Source: CAD feature listing. Evaluate the final solid. Frame: model axes, mm. Face numbers are marked on the shaded views. A direction names the side the tool comes from. Coordinates: 2 decimals unless noted, no trailing zeros. Loops run counter-clockwise (first coordinate to the right, second up) from the corner with the lowest first, then second, coordinate; pieces in that order, holes last. Notation, with made-up numbers: (12.25, -10.5) -> (64.25, -10.5) arc R15 ccw to (64.25, 11.5) -> close; hole circle Ø1 at (21.25, -32.75). An arc over 180 degrees is marked (long way). Answer as a JSON object with one key per item and string values. Group by question number.
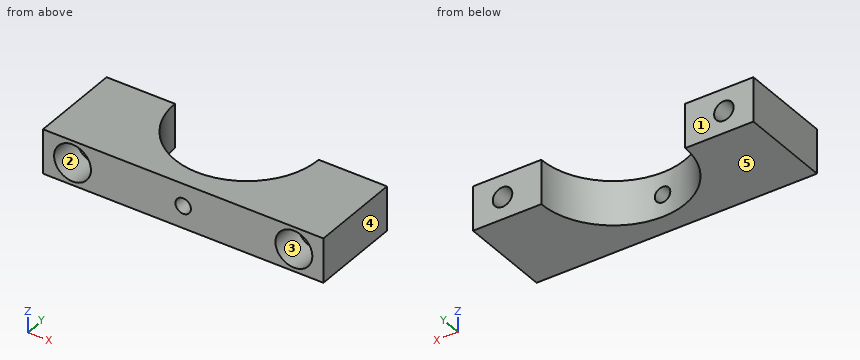
from build123d import *

# Parameters (mm, degrees)
SKETCH_1_W                = 76
SKETCH_1_H                = 12
EXTRUDE_1_DEPTH           = 25
CUT_EXTRUDE_1_REACH       = 49.043
SKETCH_2_R                = 19.5
HOLE_WIZARD_M5_1_D        = 4.2
HOLE_WIZARD_1_D           = 5.3
HOLE_WIZARD_1_CBORE_D     = 10
HOLE_WIZARD_1_CBORE_DEPTH = 8.7


with BuildPart() as part:
    # 草图1 → 凸台-拉伸1 (new body)
    with BuildSketch(Plane(origin=(0, 0, 0), x_dir=(1, 0, 0), z_dir=(0, 1, 0))):
        Rectangle(SKETCH_1_W, SKETCH_1_H)
    extrude(amount=-EXTRUDE_1_DEPTH)

    # 草图2 → 切除-拉伸1 (cut, up to next)
    with BuildSketch(Plane.XY.offset(6), mode=Mode.PRIVATE) as cut_extrude_1_sk1:
        Circle(SKETCH_2_R)
    cut_extrude_1_tool1 = extrude(cut_extrude_1_sk1.sketch, amount=-CUT_EXTRUDE_1_REACH, mode=Mode.PRIVATE) & part.part
    add(cut_extrude_1_tool1.solids().sort_by_distance((0, 0, 6))[0], mode=Mode.SUBTRACT)

    # M5 螺纹孔1 (through all)
    with Locations(Plane.XZ.offset(25)):
        with Locations((0, 0)):
            Hole(HOLE_WIZARD_M5_1_D / 2)

    # 打孔尺寸根据内六角圆柱头螺钉的类型1 (through all)
    with Locations(Plane.XZ.offset(25)):
        with Locations((-30, 0), (30, 0)):
            CounterBoreHole(HOLE_WIZARD_1_D / 2, HOLE_WIZARD_1_CBORE_D / 2, HOLE_WIZARD_1_CBORE_DEPTH)


solid = part.part
1. Section query C-C on y = -3.5. Return loops of the section in (x, z).
2. Reachability of the marked faces 1 and 2 from +Z, -Z, +X, -X, +Y, -Y: full face, straight path, thin tool, end or side. Return the list, or none.
3. Section query A-A on x = 30. Return loops of the section in (y, z).
4. Section query D-D on y = -14.25. Return loops of the section in (x, z), then the cut area to 3 significant figures.
5. Mould query, pull axis Z, two halves, no side actions, for the marked faces 3, 4 and 5. Classes: pulls with the +Z half, pulls with the -Z half, needs draft (parallel to the pull), parting line crosses it, or undercut.
6. Section query B-B on z = 0. Return loops of the section in (x, y).
7. Ray query, L1, parallel to Z at x = -30, y = -11; L2, parallel to X at y = -12.75, z = 0.25; L3, parallel to X at y = -10.75, z = -2.25. Return the intervals inside material, ascending.
8. Pin query (flat end, axial travel): pin 1 Ø6.5 at (x, z) = (0, 0) entering from +Y; pin 2 Ø5 at (x, z) = (31.5, 1) entering from -Y. Return the tip coordinate at first contact, or that it passes through.
Solved:
{
 "1": {"outline": "(-38, -6) -> (-19.18, -6) -> (-19.18, 6) -> (-38, 6) -> close; (19.18, -6) -> (38, -6) -> (38, 6) -> (19.18, 6) -> close; hole circle Ø5.3 at (-30, 0); hole circle Ø5.3 at (30, 0)"},
 "2": {"face 1": "+Z, -Z, +X, -X, +Y", "face 2": "-Y"},
 "3": {"outline": "(-25, -6) -> (0, -6) -> (0, -2.65) -> (-16.3, -2.65) -> (-16.3, -5) -> (-25, -5) -> close; (-25, 5) -> (-16.3, 5) -> (-16.3, 2.65) -> (0, 2.65) -> (0, 6) -> (-25, 6) -> close"},
 "4": {"outline": "(-38, -6) -> (-13.31, -6) -> (-13.31, 6) -> (-38, 6) -> close; (13.31, -6) -> (38, -6) -> (38, 6) -> (13.31, 6) -> close; hole circle Ø5.3 at (-30, 0); hole circle Ø5.3 at (30, 0)", "area": "548 mm^2"},
 "5": {"face 3": "undercut", "face 4": "needs draft", "face 5": "pulls with the -Z half"},
 "6": {"outline": "(-38, -25) -> (-35, -25) -> (-35, -16.3) -> (-32.65, -16.3) -> (-32.65, 0) -> (-38, 0) -> close; (-27.35, -16.3) -> (-25, -16.3) -> (-25, -25) -> (-2.1, -25) -> (-2.1, -19.39) arc R19.5 cw to (-19.5, 0) -> (-27.35, 0) -> close; (2.1, -25) -> (25, -25) -> (25, -16.3) -> (27.35, -16.3) -> (27.35, 0) -> (19.5, 0) arc R19.5 cw to (2.1, -19.39) -> close; (32.65, -16.3) -> (35, -16.3) -> (35, -25) -> (38, -25) -> (38, 0) -> (32.65, 0) -> close"},
 "7": {"L1": "-6 to -2.65, 2.65 to 6", "L2": "-38 to -32.64, -27.36 to -14.75, 14.75 to 27.36, 32.64 to 38", "L3": "-38 to -31.4, -28.6 to -16.27, 16.27 to 28.6, 31.4 to 38"},
 "8": {"pin 1": "y = -19.23", "pin 2": "y = -16.3"}
}
